```python
from build123d import *

# Parameters (mm, degrees)
SKETCH1_R              = 4
SKETCH1_R_2            = 1.5
BASE_SIZE_DEPTH        = 4
SKETCH2_R              = 3.65
SKETCH2_R_2            = 2.15
BEARING_FEATURES_DEPTH = 0.3


with BuildPart() as part:
    # Sketch1 → Base size (new body)
    with BuildSketch(Plane(origin=(0, 0, 0), x_dir=(1, 0, 0), z_dir=(0, 1, 0))):
        with Locations(Location((0, 0, 0), (0, 0, 270))):
            Circle(SKETCH1_R)
        with Locations(Location((0, 0, 0), (0, 0, 270))):
            Circle(SKETCH1_R_2, mode=Mode.SUBTRACT)
    extrude(amount=BASE_SIZE_DEPTH)

    # Sketch2 → Bearing features (cut)
    with BuildSketch(Plane(origin=(0, 4, 0), x_dir=(1, 0, 0), z_dir=(0, 1, 0))):
        with Locations(Location((0, 0, 0), (0, 0, 270))):
            Circle(SKETCH2_R)
        with Locations(Location((0, 0, 0), (0, 0, 270))):
            Circle(SKETCH2_R_2, mode=Mode.SUBTRACT)
    bearing_features = extrude(amount=-BEARING_FEATURES_DEPTH, mode=Mode.SUBTRACT)

    # Mirror1: Bearing features across plane
    add(bearing_features.mirror(Plane.ZX.offset(2)), mode=Mode.SUBTRACT)


solid = part.part
```
Geometry check sheet. Reference: the model listing, model coordinates, mm. A direction names the side the tool comes from. Coordinates: 2 decimals unless noted, no trailing zeros. Loops run counter-clockwise (first coordinate to the right, second up) from the corner with the lowest first, then second, coordinate; pieces in that order, holes last. Notation, with made-up numbers: (80, 10) - (115, 10) arc R24 ccw to (115, 45) - close; hole circle Ø2 at (23.5, 55). An arc over 180 degrees is marked (long way). One line per item, written item: value. Start each with the question number.
(1) Cross-section at D-D on z = 2.5. Enter the section's corners in (x, y).
(2) Tool access check on faces 1 (the flat face through (-2, 0.3, 2)), 2 (the cylindrical face through (0.45, 1.97, 1.43)). Record the directions out of +Z, -Z, +X, -X, +Y, -Y that give a thin tool (end or side, any length) a straight path to the whole face; none if there is none.
(3) Mould release check, pull along X, two halves, no side actions. Record for faces 3 (the flat face through (-2, 3.7, 2)), 4 (the flat face through (-1.4, 4, 0.9)), 5 (the cylindrical face through (-3.905, 1.972, -0.867)): released by +X, released by -X, zero draft, split by the parting line, or undercut.
(4) Cross-section at A-A on z = 0. Enter the section's corners in (x, y), plus the area to 3 significant figures.
(5) Cross-section at C-C on y = 0.7. Enter the section's corners in (x, z).
(6) Material ranges on line 1 (X direction, y = 0.1, z = 0); line 2 (X direction, y = 2.75, z = 0); line 3 (Y direction, x = 2, z = -1), recorded low to high. Write a range as [from, to].
(7) Depth check by flat-ended pin: P1, Ø1, axis at y = 1.5, z = 1.5, coming from the -X side. Enter the tip coordinate at first touch or a pass-through.
(8) Cross-section at B-B on x = 0. Enter the section's corners in (y, z).
Results below:
1. outline: (-3.12, 0) - (-2.66, 0) - (-2.66, 0.3) - (2.66, 0.3) - (2.66, 0) - (3.12, 0) - (3.12, 4) - (2.66, 4) - (2.66, 3.7) - (-2.66, 3.7) - (-2.66, 4) - (-3.12, 4) - close
2. face 1: -Y
2. face 2: +Y, -Y
3. face 3: undercut
3. face 4: zero draft
3. face 5: split by the parting line
4. outline: (-4, 0) - (-3.65, 0) - (-3.65, 0.3) - (-2.15, 0.3) - (-2.15, 0) - (-1.5, 0) - (-1.5, 4) - (-2.15, 4) - (-2.15, 3.7) - (-3.65, 3.7) - (-3.65, 4) - (-4, 4) - close; (1.5, 0) - (2.15, 0) - (2.15, 0.3) - (3.65, 0.3) - (3.65, 0) - (4, 0) - (4, 4) - (3.65, 4) - (3.65, 3.7) - (2.15, 3.7) - (2.15, 4) - (1.5, 4) - close
4. area: 18.2 mm2
5. outline: circle Ø8 at (0, 0); hole circle Ø3 at (0, 0)
6. line 1: x = [-4, -3.65], [-2.15, -1.5], [1.5, 2.15], [3.65, 4]
6. line 2: x = [-4, -1.5], [1.5, 4]
6. line 3: y = [0.3, 3.7]
7. P1: stops at x = -3.87
8. outline: (0, -4) - (4, -4) - (4, -3.65) - (3.7, -3.65) - (3.7, -2.15) - (4, -2.15) - (4, -1.5) - (0, -1.5) - (0, -2.15) - (0.3, -2.15) - (0.3, -3.65) - (0, -3.65) - close; (0, 1.5) - (4, 1.5) - (4, 2.15) - (3.7, 2.15) - (3.7, 3.65) - (4, 3.65) - (4, 4) - (0, 4) - (0, 3.65) - (0.3, 3.65) - (0.3, 2.15) - (0, 2.15) - close
